Part model, mm, in its own coordinate system. A direction names the side the tool comes from. Round coordinates to 2 decimals unless told otherwise and drop trailing zeros. Order: outer loops, then holes, each group sorted by start corner. A loop starts at its lowest first (then second) coordinate and runs counter-clockwise, first axis right, second up. Notation, with made-up numbers: (49.25, 9) -> (107.25, 9) arc R19 cw to (107.25, 21) -> close; hole circle Ø3 at (24, 18). An arc over 180 degrees is marked (long way). Return JSON: item names as keys, results as strings. Group by question number.
from build123d import *

# Parameters (mm, degrees)
SKETCH1_W     = 20
SKETCH1_H     = 5
SCALE_1_SCALE = 0.6


with BuildPart() as part:
    # Sketch1 → Revolve2 (revolve)
    with BuildSketch(Plane.XY, mode=Mode.PRIVATE) as revolve2_sk:
        with Locations((10, -29.5)):
            Rectangle(SKETCH1_W, SKETCH1_H)
        with BuildLine():
            Line((7.5, 0), (0, 0))
            Line((0, 0), (0, -27))
            Line((0, -27), (20, -27))
            ThreePointArc((20, -27), (10.738142241, -14.894378592), (7.5, 0))
        make_face()
        with BuildLine():
            ThreePointArc((8.747613634, 8.812516428), (8.61554983, 18.734698905), (0, 23.658056202))
            Line((0, 23.658056202), (0, 3.658056202))
            Line((0, 3.658056202), (7.5, 3.658056202))
            ThreePointArc((7.5, 3.658056202), (7.775883858, 6.319499484), (8.747613634, 8.812516428))
        make_face()
        Polygon((7.5, 3.658056202), (0, 3.658056202), (0, 0), (7.5, 0), (10, 0), (10, 3.658056202), align=None)
    revolve(revolve2_sk.sketch.rotate(Axis((0, 36.358430306, 0), (0, -1, 0)), 90), axis=Axis((0, 36.358430306, 0), (0, -1, 0)))


with BuildPart() as part_1:
    # 缩放比例1: scaled about (0, 0, 0)
    add(part.part.scale(SCALE_1_SCALE))


solid = part_1.part
(1) Saw through at B-B, the plane z = 0. List the corners of the cut face in (x, y), and give its area (3 significant figures).
(2) Saw through at C-C, the plane y = -14. List the corners of the cut face in (x, z), and give its area (3 significant figures).
(3) Probe L1, parallel to Y at x = 3.75, z = -4; L2, parallel to Y at x = -8.5, z = -5.75; L3, parallel to Y at x = 10.25, z = 2. List the from-to ranges inside material, lowest first. Write a range as [from, to].
(4) Pin check, flat tips, straight feed: P1, Ø6, axis at x = 3, z = 7, coming from the +Y side; P2, Ø10, axis at x = 6, z = -3, coming from the +Y side; P3, Ø3, axis at y = 10, z = -0.5, coming from the +X side. Stop position of each tip, or through.
(5) Saw through at D-D, the plane y = 8.5. List the corners of the cut face in (x, z).
(6) Saw through at A-A, the plane x = 0. List the corners of the cut face in (y, z).
(7) Mould opens along Y. For faces 3 (the cylindrical face through (-3.604, -17.679, 11.446)), 4 (the flat face through (0, -19.2, 0)), 5 (the flat face through (-4.5, 0, 1.4)) say: pulls with the +Y half, pulls with the -Y half, needs draft (parallel to the pull), parting line crosses it, or undercut.
(8) Tool access for faces 1 (the flat face through (-4.5, 2.195, -1.4)), 2 (the cylindrical face through (-1.802, 1.113, 5.723)): list every direction of +Z, -Z, +X, -X, +Y, -Y with a clear straight run to the whole face (end or side of a thin tool).
Results are:
{
 "1": {"outline": "(-12, -19.2) -> (12, -19.2) -> (12, -16.2) arc R21 cw to (4.5, 0) -> (6, 0) -> (6, 2.19) -> (4.5, 2.19) arc R6 cw to (5.25, 5.29) arc R6 ccw (long way) to (-5.25, 5.29) arc R6 cw to (-4.5, 2.19) -> (-6, 2.19) -> (-6, 0) -> (-4.5, 0) arc R21 cw to (-12, -16.2) -> close", "area": "437 mm^2"},
 "2": {"outline": "circle Ø19.49 at (0, 0)", "area": "298 mm^2"},
 "3": {"L1": "y = [-19.2, -6.46], [0, 2.19], [5.76, 10.63]", "L2": "y = [-19.2, -14.56]", "L3": "y = [-19.2, -14.75]"},
 "4": {"P1": "stops at y = 12.03", "P2": "stops at y = 13.95", "P3": "stops at x = 5.99"},
 "5": {"outline": "circle Ø11.98 at (0, 0)"},
 "6": {"outline": "(-19.2, -12) -> (-16.2, -12) arc R21 cw to (0, -4.5) -> (0, -6) -> (2.19, -6) -> (2.19, -4.5) arc R6 cw to (5.29, -5.25) arc R6 ccw (long way) to (5.29, 5.25) arc R6 cw to (2.19, 4.5) -> (2.19, 6) -> (0, 6) -> (0, 4.5) arc R21 cw to (-16.2, 12) -> (-19.2, 12) -> close"},
 "7": {"face 3": "needs draft", "face 4": "pulls with the -Y half", "face 5": "undercut"},
 "8": {"face 1": "none", "face 2": "+Y"}
}
